from build123d import *

# Parameters (mm, degrees)
SKETCH1_W               = 15
SKETCH1_H               = 22
BOSS_EXTRUDE1_DEPTH     = 8
SKETCH2_R               = 5.25
CUT_EXTRUDE1_DEPTH      = 6
CUT_EXTRUDE2_REACH      = 24.694
CUT_EXTRUDE2_END_RADIUS = 5.25
SKETCH3_W               = 6
SKETCH3_H               = 3.2
SKETCH4_W               = 13
SKETCH4_H               = 1.5
CUT_EXTRUDE3_DEPTH      = 10
SKETCH5_R               = 0.8
CUT_EXTRUDE4_DEPTH      = 20.544820286
CUT_EXTRUDE5_DEPTH      = 21.248456731
FILLET1_R               = 1


with BuildPart() as part:
    # Sketch1 → Boss-Extrude1 (new body)
    with BuildSketch(Plane(origin=(0, 0, -7.5), x_dir=(0, 0, 1), z_dir=(-1, 0, 0))):
        Rectangle(SKETCH1_W, SKETCH1_H)
    extrude(amount=BOSS_EXTRUDE1_DEPTH)

    # Sketch2 → Cut-Extrude1 (cut)
    with BuildSketch(Plane.ZY.offset(8)):
        with Locations((-7.5, 0)):
            Circle(SKETCH2_R)
    extrude(amount=-CUT_EXTRUDE1_DEPTH, mode=Mode.SUBTRACT)

    # Cut-Extrude2: up to this cylinder (the profile starts outside it)
    cut_extrude2_end = Plane(origin=(-5, 0, -7.5), z_dir=(-1, 0, 0)) * Cylinder(CUT_EXTRUDE2_END_RADIUS, 60.888, mode=Mode.PRIVATE)
    # Sketch3 → Cut-Extrude2 (cut, up to the surface)
    with BuildSketch(Plane(origin=(5, 0, 0), x_dir=(1, 0, 0), z_dir=(0, 0, 1)), mode=Mode.PRIVATE) as cut_extrude2_sk1:
        with Locations((-10, 0)):
            Rectangle(SKETCH3_W, SKETCH3_H)
    cut_extrude2_tool1 = extrude(cut_extrude2_sk1.sketch, amount=-CUT_EXTRUDE2_REACH, mode=Mode.PRIVATE) - cut_extrude2_end
    add(cut_extrude2_tool1.solids().sort_by_distance((-5, 0, 0))[0], mode=Mode.SUBTRACT)

    # Sketch4 → Cut-Extrude3 (cut)
    with BuildSketch(Plane(origin=(0, 0, 0), x_dir=(0, 0, -1), z_dir=(1, 0, 0))):
        with Locations((7.5, 8.75)):
            Rectangle(SKETCH4_W, SKETCH4_H)
        with Locations((7.5, -8.75)):
            Rectangle(SKETCH4_W, SKETCH4_H)
    extrude(amount=-CUT_EXTRUDE3_DEPTH, mode=Mode.SUBTRACT)

    # Sketch5 → Cut-Extrude4 (cut, through all)
    with BuildSketch(Plane.ZY.offset(2)):
        with Locations((-7.5, 0)):
            Circle(SKETCH5_R)
    extrude(amount=-CUT_EXTRUDE4_DEPTH, mode=Mode.SUBTRACT)

    # Sketch6 → Cut-Extrude5 (cut, through all)
    with BuildSketch(Plane.XY):
        Polygon((0, -11), (-6.5, -11), (0, -5.545852397), align=None)
        Polygon((0, 11), (-6.5, 11), (0, 5.545852397), align=None)
    extrude(amount=-CUT_EXTRUDE5_DEPTH, mode=Mode.SUBTRACT)

    # Fillet1
    fillet1_edges = [part.edges().sort_by_distance(p)[0] for p in [
        (-8, 0, -12.75),
        (-8, 1.6, -1.249875003),
        (-8, -1.6, -1.249875003),
    ]]
    fillet(fillet1_edges, radius=FILLET1_R)


solid = part.part
The listing builds one solid part. Answer for the finished solid, in the listing's coordinates (mm). A direction names the side the tool comes from. Coordinates: 2 decimals unless noted, no trailing zeros. Order: outer loops, then holes, each group sorted by start corner. A loop starts at its lowest first (then second) coordinate and runs counter-clockwise, first axis right, second up.
Q1. A cutting plane is placed at C-C, the plane x = -3.5. Write down the section's boundary in (y, z).
Q2. Which of the six approach directions +Z, -Z, +X, -X, +Y, -Y give full straight-line access (tool end or side, diameter ignored) to faces 1 (the face through (-2, 0, -6)), 2 (the face through (-6, -9.5, -7)), 3 (the face through (-5, 1.6, -1))?
Q3. Consider line 1 (Y direction, x = -6, z = -11.5); line 2 (Y direction, x = -3.9, z = -7.5); line 3 (Y direction, x = -7.25, z = -12). Determine where each line is inside the solid, lowest interval first.
Q4. A cutting plane is placed at B-B, the plane z = -7.5. Write down the section's boundary in (x, y).
Q5. Given P1, Ø1.2, axis at x = -5.5, z = -1, coming from the +Y side; P2, Ø1.2, axis at x = -5, z = -1.5, coming from the -Y side; P3, Ø8.5, axis at y = 1.5, z = -7.5, coming from the -X side; P4, Ø1.3, axis at y = 0, z = -7.5, coming from the +X side, each flat-ended and moving along its own axis, determine where each tip first touches the part or whether it passes through.
Q6. A cutting plane is placed at A-A, the plane y = 0. Write down the section's boundary in (x, z).
Q7. For a pull along Z with two mould halves and no side action, classify faces 4 (the face through (-4, 2, 0)), 5 (the face through (-2.573, -7.705, -7.395)), 6 (the face through (-6, 9.5, -7)), 7 (the face through (-1, 0, -8.3)) as pulls with the +Z half, pulls with the -Z half, needs draft (parallel to the pull), parting line crosses it, or undercut.
Q8. A cutting plane is placed at D-D, the plane z = -4. State how many separate pieces and enclosed holes the cut face has, and give its area (3 significant figures).
Answers follow:
1. outline: (-8.48, -15) - (8.48, -15) - (8.48, -14) - (8, -14) - (8, -1) - (8.48, -1) - (8.48, 0) - (1.6, 0) - (1.6, -2.5) arc R5.25 cw (long way) to (-1.6, -2.5) - (-1.6, 0) - (-8.48, 0) - (-8.48, -1) - (-8, -1) - (-8, -14) - (-8.48, -14) - close
2. face 1: -X
2. face 2: +X, -X
2. face 3: +Z, -X
3. line 1: y = -10.58 to -9.5, -8 to -3.4, 3.4 to 8, 9.5 to 10.58
3. line 2: y = -8 to -5.25, 5.25 to 8
3. line 3: y = -11 to -9.5, -8 to -2.77, 2.77 to 8, 9.5 to 11
4. outline: (-8, -11) - (-6.5, -11) - (-4.71, -9.5) - (-8, -9.5) - close; (-8, -8) - (-2.92, -8) - (0, -5.55) - (0, -0.8) - (-2, -0.8) - (-2, -5.25) - (-7, -5.25) arc R1 ccw to (-8, -6.25) - close; (-8, 6.25) arc R1 ccw to (-7, 5.25) - (-2, 5.25) - (-2, 0.8) - (0, 0.8) - (0, 5.55) - (-2.92, 8) - (-8, 8) - close; (-8, 9.5) - (-4.71, 9.5) - (-6.5, 11) - (-8, 11) - close
5. P1: stops at y = 10.66
5. P2: stops at y = -10.24
5. P3: stops at x = -7.87
5. P4: passes through
6. outline: (-8, -15) - (0, -15) - (0, -8.3) - (-2, -8.3) - (-2, -12.75) - (-7, -12.75) arc R1 ccw to (-8, -13.75) - close; (-2, -6.7) - (0, -6.7) - (0, 0) - (-2, 0) - close
7. face 4: pulls with the +Z half
7. face 5: needs draft
7. face 6: undercut
7. face 7: undercut
8. separate pieces: 3
8. enclosed holes: 0
8. area: 80.5 mm2
